Verification items for this drawing (mm, ordinates from the low corner). A direction names the side the tool comes from. Coordinates: 2 decimals unless noted, no trailing zeros. Order: outer loops, then holes, each group sorted by start corner. A loop starts at its lowest first (then second) coordinate and runs counter-clockwise, first axis right, second up. Notation, with made-up numbers: M 66,52 L 102,52 A14 ccw 102,72 Z; hole C -12.5,-34 d5. An arc over 180 degrees is marked long. Return JSON: item names as keys, results as strings. Group by question number.
1. Gauge pin test, flat ends, axial feed: pin 1 (1.5 mm diameter, centred on y = 5, z = 19.5, fed in from +X); pin 2 (5 mm diameter, centred on y = 10.5, z = 25, fed in from +X); pin 3 (1.4 mm diameter, centred on x = 40, y = 7.5, fed in from +Z); pin 4 (4 mm diameter, centred on x = 25, y = 3, fed in from -Z). Record the tip position at first contact, or that the pin passes through.
2. Section check C-C, the plane x = 40. Record the cut outline in (y, z).
3. Section check B-B, the plane y = 7.5. Record the cut outline in (x, z), plus the area to 3 significant figures.
4. Mould release check, pull along Z, two halves, no side actions. Record for the marked faces 1, 2 and 3: +Z half, -Z half, draft (parallel to the pull), parting line (faces both ways), or undercut.
5. Section check D-D, the plane z = 26. Record the cut outline in (x, y), plus the area to 3 significant figures.
6. Material ranges on line 1 along Y through (x, z) = (20, 23); line 2 along X through (y, z) = (7.5, 22); line 3 along Y through (x, z) = (40, 22), recorded low to high.
7. Set-up check for the marked faces 4 and 5: record each of +Z, -Z, +X, -X, +Y, -Y from which the full face is reachable in a straight line by a thin tool's end or side.
8. Section check A-A, the plane y = 13. Record the cut outline in (x, z).
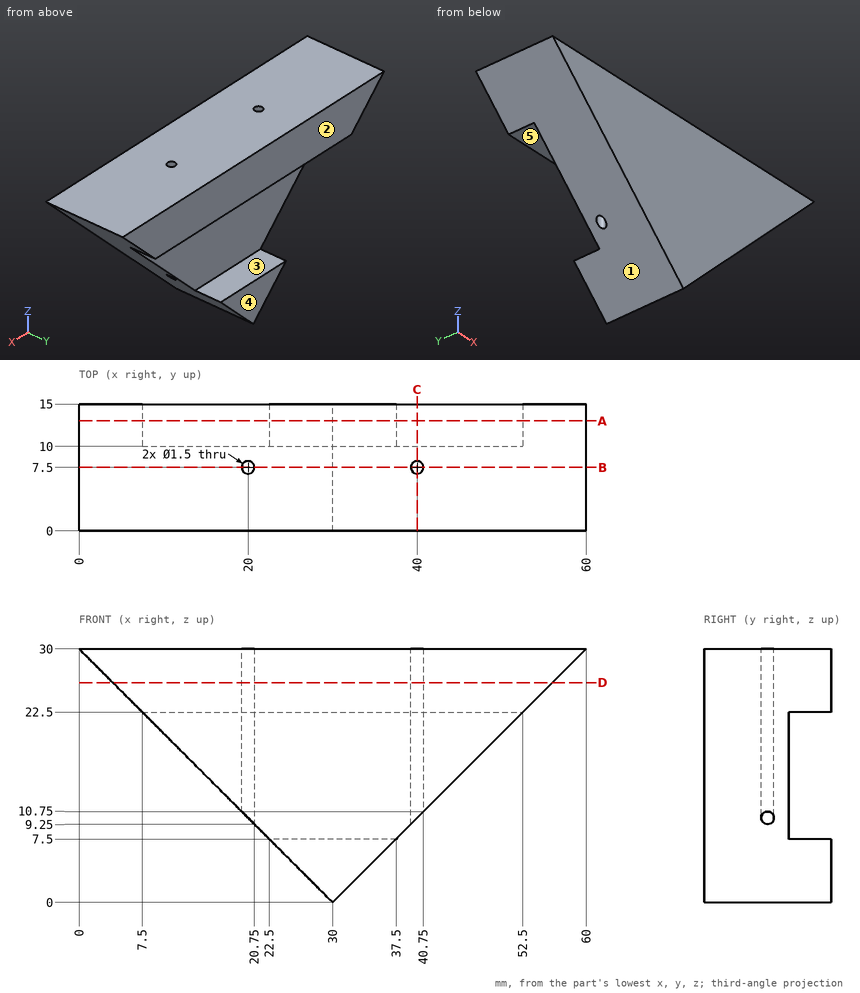
Answers follow:
{
 "1": {"pin 1": "x = 50.25", "pin 2": "x = 57.5", "pin 3": "through", "pin 4": "z = 3"},
 "2": {"outline": "M 0,10 L 6.75,10 L 6.75,30 L 0,30 Z; M 8.25,10 L 10,10 L 10,22.5 L 15,22.5 L 15,30 L 8.25,30 Z"},
 "3": {"outline": "M 0,30 L 19.25,10.75 L 19.25,30 Z; M 20.75,9.25 L 30,0 L 39.25,9.25 L 39.25,30 L 20.75,30 Z; M 40.75,10.75 L 60,30 L 40.75,30 Z", "area": "840 mm^2"},
 "4": {"face 1": "-Z half", "face 2": "draft", "face 3": "undercut"},
 "5": {"outline": "M 4,0 L 56,0 L 56,15 L 4,15 Z; hole C 20,7.5 d1.5; hole C 40,7.5 d1.5", "area": "776 mm^2"},
 "6": {"line 1": "0 to 6.75, 8.25 to 15", "line 2": "8 to 19.25, 20.75 to 39.25, 40.75 to 52", "line 3": "0 to 6.75, 8.25 to 10"},
 "7": {"face 4": "+Z, -Z, +X, -X, +Y", "face 5": "+X, -X, +Y"},
 "8": {"outline": "M 0,30 L 7.5,22.5 L 52.5,22.5 L 60,30 Z; M 22.5,7.5 L 30,0 L 37.5,7.5 Z"}
}
